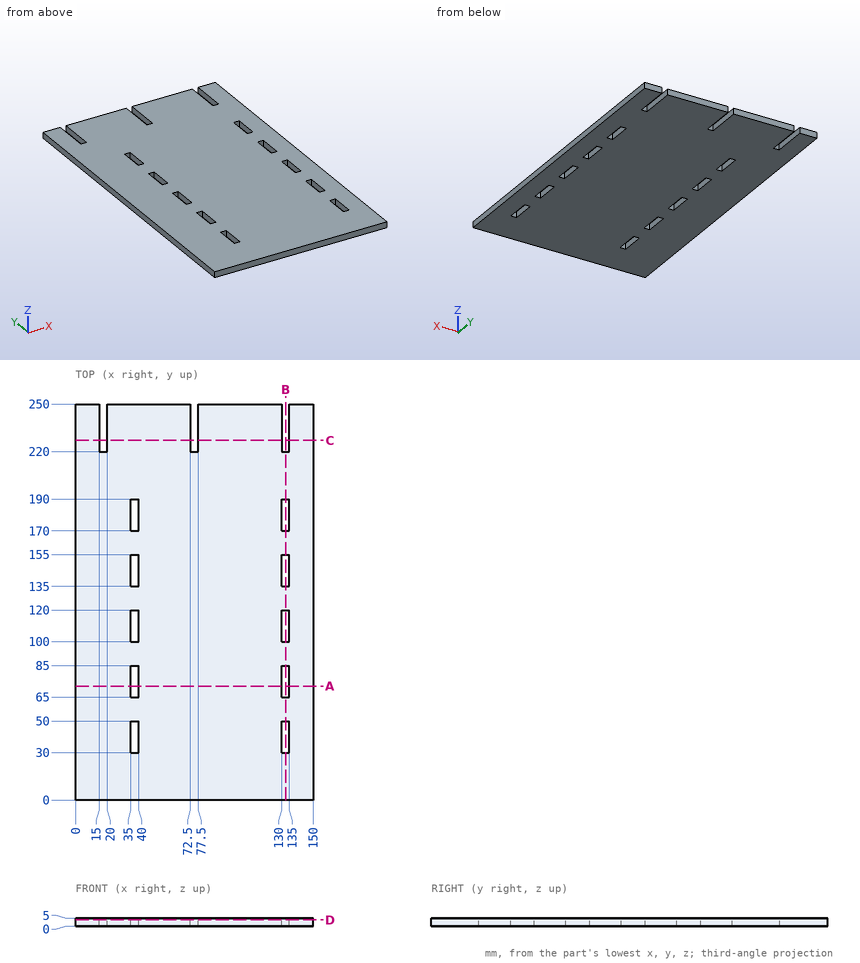
The figure shows three views and two pictorial views of one solid part (mm, origin at its lowest corner). Answer the questions. Coordinates: 2 decimals unless noted, no trailing zeros. Order: outer loops, then holes, each group sorted by start corner. A loop starts at its lowest first (then second) coordinate and runs counter-clockwise, first axis right, second up.
Q1. A cutting plane is placed at C-C, the plane y = 227. Write down the section's boundary in (x, z).
Q2. Consider line 1 (X direction, y = 79, z = 3.9); line 2 (Y direction, x = 39.5, z = 2.4); line 3 (Y direction, x = 73, z = 4.5). Determine where each line is inside the solid, lowest interval first.
Q3. A cutting plane is placed at D-D, the plane z = 4. State how many separate pieces and enclosed holes the cut face has, and give its area (4 significant figures).
Q4. A cutting plane is placed at B-B, the plane x = 132.5. Write down the section's boundary in (y, z).
Q5. A cutting plane is placed at A-A, the plane y = 72. Write down the section's boundary in (x, z), and give its area (3 significant figures).
Answers follow:
1. outline: (0, 0) - (15, 0) - (15, 5) - (0, 5) - close; (20, 0) - (72.5, 0) - (72.5, 5) - (20, 5) - close; (77.5, 0) - (130, 0) - (130, 5) - (77.5, 5) - close; (135, 0) - (150, 0) - (150, 5) - (135, 5) - close
2. line 1: x = 0 to 35, 40 to 130, 135 to 150
2. line 2: y = 0 to 30, 50 to 65, 85 to 100, 120 to 135, 155 to 170, 190 to 250
2. line 3: y = 0 to 220
3. separate pieces: 1
3. enclosed holes: 10
3. area: 36,050 mm2
4. outline: (0, 0) - (30, 0) - (30, 5) - (0, 5) - close; (50, 0) - (65, 0) - (65, 5) - (50, 5) - close; (85, 0) - (100, 0) - (100, 5) - (85, 5) - close; (120, 0) - (135, 0) - (135, 5) - (120, 5) - close; (155, 0) - (170, 0) - (170, 5) - (155, 5) - close; (190, 0) - (220, 0) - (220, 5) - (190, 5) - close
5. outline: (0, 0) - (35, 0) - (35, 5) - (0, 5) - close; (40, 0) - (130, 0) - (130, 5) - (40, 5) - close; (135, 0) - (150, 0) - (150, 5) - (135, 5) - close
5. area: 700 mm2
